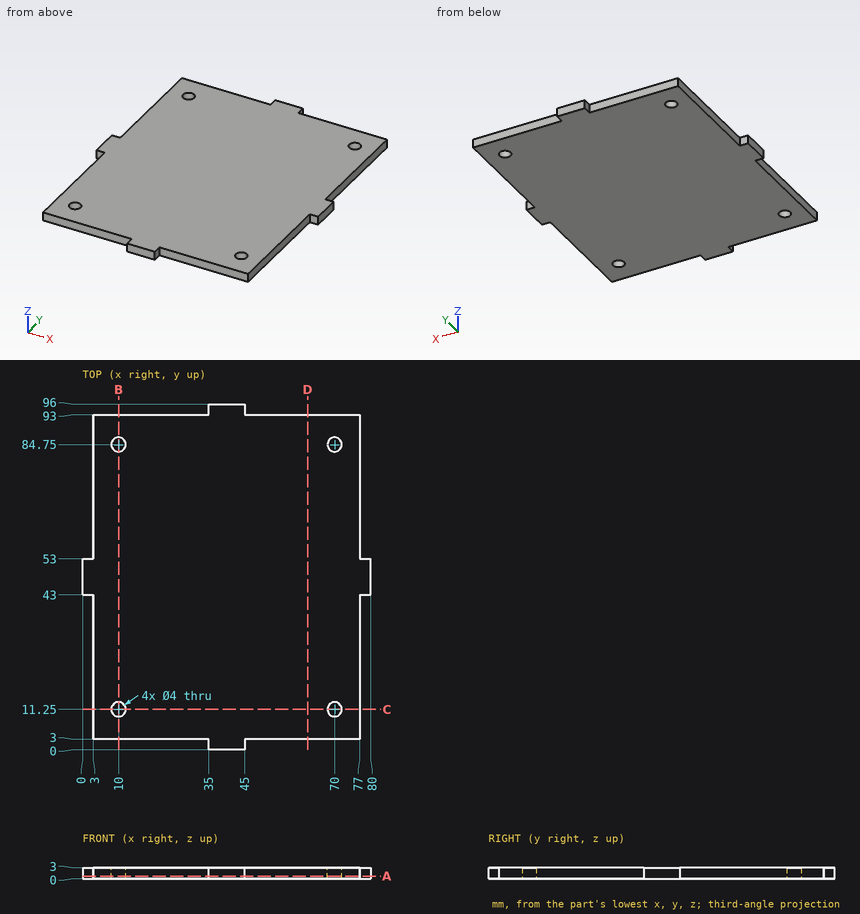
Geometry check sheet. Reference: drawing and pictorial views, mm from the part's lowest x, y, z. Coordinates: 2 decimals unless noted, no trailing zeros. Order: outer loops, then holes, each group sorted by start corner. A loop starts at its lowest first (then second) coordinate and runs counter-clockwise, first axis right, second up.
1. Sectioned sample at B-B, the plane x = 10. Record the cut outline in (y, z).
Results found:
outline: (3, 0) - (9.25, 0) - (9.25, 3) - (3, 3) - close; (13.25, 0) - (82.75, 0) - (82.75, 3) - (13.25, 3) - close; (86.75, 0) - (93, 0) - (93, 3) - (86.75, 3) - close
2. Go/stop test with flat-tipped pins: pin 1 Ø0.9 at (x, z) = (64.5, 1) entering from +Y; pin 2 Ø1.5 at (y, z) = (79.5, 2) entering from +X; pin 3 Ø0.9 at (x, z) = (58.5, 1.5) entering from -Y. Record where each tip stops, or that it passes through.
Results found:
pin 1: stops at y = 93
pin 2: stops at x = 77
pin 3: stops at y = 3
3. Sectioned sample at C-C, the plane y = 11.25. Record the cut outline in (x, z), and give its area (3 significant figures).
Results found:
outline: (3, 0) - (8, 0) - (8, 3) - (3, 3) - close; (12, 0) - (68, 0) - (68, 3) - (12, 3) - close; (72, 0) - (77, 0) - (77, 3) - (72, 3) - close
area: 198 mm2
4. Sectioned sample at A-A, the plane z = 0.7. Record the cut outline in (x, y), and give its area (3 significant figures).
Results found:
outline: (0, 43) - (3, 43) - (3, 3) - (35, 3) - (35, 0) - (45, 0) - (45, 3) - (77, 3) - (77, 43) - (80, 43) - (80, 53) - (77, 53) - (77, 93) - (45, 93) - (45, 96) - (35, 96) - (35, 93) - (3, 93) - (3, 53) - (0, 53) - close; hole circle Ø4 at (10, 11.25); hole circle Ø4 at (10, 84.75); hole circle Ø4 at (70, 11.25); hole circle Ø4 at (70, 84.75)
area: 6,730 mm2
5. Sectioned sample at D-D, the plane x = 62.5. Record the cut outline in (y, z), and give its area (3 significant figures).
Results found:
outline: (3, 0) - (93, 0) - (93, 3) - (3, 3) - close
area: 270 mm2
6. Scan lines: line 1 (Y direction, x = 70, z = 0.75); line 2 (X direction, y = 11.5, z = 0.9); line 3 (X direction, y = 24.5, z = 1.15). Record each from-to range of solid material in increasing order.
Results found:
line 1: y = 3 to 9.25, 13.25 to 82.75, 86.75 to 93
line 2: x = 3 to 8.02, 11.98 to 68.02, 71.98 to 77
line 3: x = 3 to 77
